Build history of the part. All positions in model axes, mm. Face numbers are marked on the shaded views. A direction names the side the tool comes from. Round coordinates to 2 decimals unless told otherwise and drop trailing zeros. Order: outer loops, then holes, each group sorted by start corner. A loop starts at its lowest first (then second) coordinate and runs counter-clockwise, first axis right, second up. Notation, with made-up numbers: (52, -7) -> (68, -7) arc R18 cw to (68, 23) -> close; hole circle Ø9 at (-6.5, 8). An arc over 180 degrees is marked (long way). Answer as a JSON object with one key per item and string values.
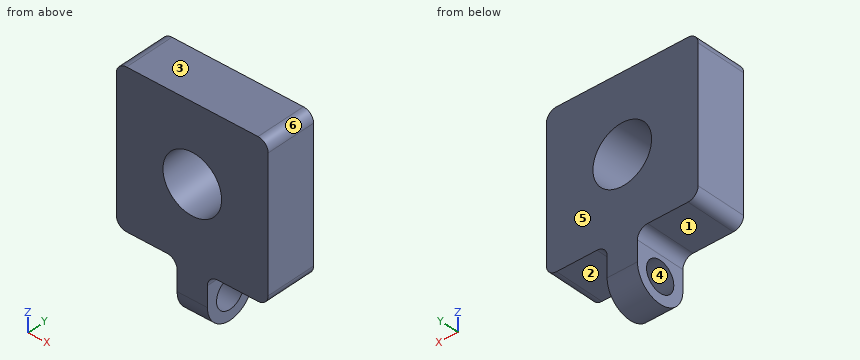
from build123d import *

# Parameters (mm, degrees)
SKETCH1_W           = 15
SKETCH1_H           = 15
BOSS_EXTRUDE1_DEPTH = 5
SKETCH3_R           = 1.5
BOSS_EXTRUDE2_DEPTH = 1.5
CUT_EXTRUDE1_REACH  = 17.819
SKETCH4_R           = 2.9
FILLET1_R           = 1


with BuildPart() as part:
    # Sketch1 → Boss-Extrude1 (new body)
    with BuildSketch(Plane(origin=(0, 0, 0), x_dir=(1, 0, 0), z_dir=(0, 1, 0))):
        Rectangle(SKETCH1_W, SKETCH1_H)
    extrude(amount=BOSS_EXTRUDE1_DEPTH)

    # Sketch3 → Boss-Extrude2 (add, symmetric)
    with BuildSketch(Plane(origin=(0, 0, 0), x_dir=(0, 0, -1), z_dir=(1, 0, 0))):
        with BuildLine():
            Line((7.5, 5), (10.5, 5))
            ThreePointArc((10.5, 5), (13, 2.5), (10.5, 0))
            Line((10.5, 0), (7.5, 0))
            Line((7.5, 0), (7.5, 5))
        make_face()
        with Locations((10.5, 2.5)):
            Circle(SKETCH3_R, mode=Mode.SUBTRACT)
    extrude(amount=BOSS_EXTRUDE2_DEPTH, both=True)

    # Sketch4 → Cut-Extrude1 (cut, up to next)
    with BuildSketch(Plane(origin=(0, 5, 0), x_dir=(1, 0, 0), z_dir=(0, 1, 0)), mode=Mode.PRIVATE) as cut_extrude1_sk1:
        with Locations(Location((0, 0, 0), (0, 0, 270))):
            Circle(SKETCH4_R)
    cut_extrude1_tool1 = extrude(cut_extrude1_sk1.sketch, amount=-CUT_EXTRUDE1_REACH, mode=Mode.PRIVATE) & part.part
    add(cut_extrude1_tool1.solids().sort_by_distance((0, 5, 0))[0], mode=Mode.SUBTRACT)

    # Fillet1
    fillet1_edges = [part.edges().sort_by_distance(p)[0] for p in [
        (1.5, 2.5, -7.5),
        (-1.5, 2.5, -7.5),
        (7.5, 2.5, 7.5),
        (-7.5, 2.5, 7.5),
        (-7.5, 2.5, -7.5),
        (7.5, 2.5, -7.5),
    ]]
    fillet(fillet1_edges, radius=FILLET1_R)


solid = part.part
1) Pull direction Z, two halves, no side cores. Call the marked faces 4, 5 and 6: pulls with the +Z half, pulls with the -Z half, needs draft (parallel to the pull), parting line crosses it, or undercut.
Checked values:
{"face 4": "undercut", "face 5": "needs draft", "face 6": "pulls with the +Z half"}
2) Cut at C-C, the plane x = 2.25. Give the cut face in (y, z).
Checked values:
{"outline": "(0, -7.53) -> (5, -7.53) -> (5, -1.83) -> (0, -1.83) -> close; (0, 1.83) -> (5, 1.83) -> (5, 7.5) -> (0, 7.5) -> close"}
3) Cut at B-B, the plane z = 0. Give the cut face in (x, y), plus the area to 3 significant figures.
Checked values:
{"outline": "(-7.5, 0) -> (-2.9, 0) -> (-2.9, 5) -> (-7.5, 5) -> close; (2.9, 0) -> (7.5, 0) -> (7.5, 5) -> (2.9, 5) -> close", "area": "46.0 mm²"}
4) Flat gauge pins, fed straight in: pin 1 Ø1.2 at (x, y) = (-4, 2.5) entering from -Z; pin 2 Ø2.5 at (y, z) = (2.5, -10.5) entering from -X. Where does each tip first touch, or does it go through?
Checked values:
{"pin 1": "stops at z = -7.5", "pin 2": "passes through"}
5) Which spindle directions (+Z, -Z, +X, -X, +Y, -Y) get a long thin tool onto all of the face, cutting with end or side? Do the marked faces 1, 2 and 3. Say none if no direction does.
Checked values:
{"face 1": "-Z, -X, +Y, -Y", "face 2": "-Z, +X, +Y, -Y", "face 3": "+Z, +X, -X, +Y, -Y"}
6) Probe L1, parallel to X at y = 3.85, z = 0; L2, parallel to Z at x = -0.25, y = 1.5; L3, parallel to Y at x = -0.7, z = -10.5. List the from-to ranges inside material, lowest first. Write a range as from..to.
Checked values:
{"L1": "x = -7.5..-2.9, 2.9..7.5", "L2": "z = -12.79..-11.62, -9.38..-2.89, 2.89..7.5", "L3": "y = 0..1, 4..5"}
7) Cut at A-A, the plane y = 2.5. Give the cut face in (x, z).
Checked values:
{"outline": "(-7.5, -6.5) arc R1 ccw to (-6.5, -7.5) -> (-2.5, -7.5) arc R1 cw to (-1.5, -8.5) -> (-1.5, -9) -> (1.5, -9) -> (1.5, -8.5) arc R1 cw to (2.5, -7.5) -> (6.5, -7.5) arc R1 ccw to (7.5, -6.5) -> (7.5, 6.5) arc R1 ccw to (6.5, 7.5) -> (-6.5, 7.5) arc R1 ccw to (-7.5, 6.5) -> close; (-1.5, -13) -> (1.5, -13) -> (1.5, -12) -> (-1.5, -12) -> close; hole circle Ø5.8 at (0, 0)"}
